CAD build for the part. Positions are in the model's coordinates, mm. Face numbers are marked on the shaded views. A direction names the side the tool comes from. Give positions to 0.01 mm unless a question says otherwise; leave off trailing zeros. Write each loop counter-clockwise with the first axis right and the second up, starting at its lowest first coordinate (ties: lowest second). Pieces come first, ordered by that corner, then holes. Notation, with made-up numbers: (60.5, 35.5) -> (93.5, 35.5) arc R22 ccw to (93.5, 73.5) -> close; hole circle Ø7 at (-30, 13). An arc over 180 degrees is marked (long way). Answer as a JSON object with one key per item and string values.
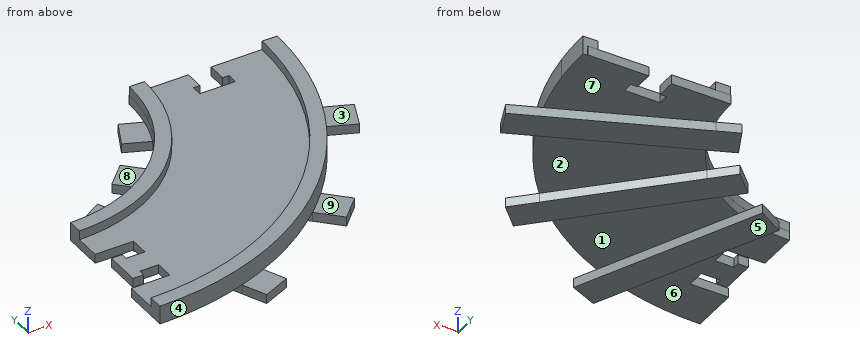
```python
from build123d import *

# Parameters (mm, degrees)
F1_DEPTH  = 3.175
F4_DEPTH  = 3.175
F6_DEPTH  = 6.35
F7_DEPTH  = 3.175
F9_DEPTH  = 25.4
F11_DEPTH = 3.175
F13_DEPTH = 3.175
F14_DEPTH = 25.4


with BuildPart() as f1:
    # F0 (on Top) → F1 (new body)
    with BuildSketch(Plane.XY):
        with BuildLine():
            Line((0, -51.2956328023), (0, -102.09075941))
            ThreePointArc((0, -102.09075941), (72.1890682753, -72.1890682753), (102.09075941, 0))
            Line((102.09075941, 0), (51.2956328023, 0))
            ThreePointArc((51.2956328023, 0), (36.2714897998, -36.2714897998), (0, -51.2956328023))
        make_face()
    extrude(amount=F1_DEPTH)

    # F3 (on face) → F4 (join)
    with BuildSketch(Plane.XY.offset(3.175)):
        with BuildLine():
            ThreePointArc((0, -56.3756328023), (39.8635922482, -39.8635922482), (56.3756328023, 0))
            Line((56.3756328023, 0), (51.3330261441, 0))
            ThreePointArc((51.3330261441, 0), (36.2979308853, -36.2979308853), (0, -51.3330261441))
            Line((0, -51.3330261441), (0, -56.3756328023))
        make_face()
        with BuildLine():
            Line((102.09075941, 0), (97.01075941, 0))
            ThreePointArc((97.01075941, 0), (68.5969658269, -68.5969658269), (0, -97.01075941))
            Line((0, -97.01075941), (0, -102.09075941))
            ThreePointArc((0, -102.09075941), (72.1890682753, -72.1890682753), (102.09075941, 0))
        make_face()
    extrude(amount=F4_DEPTH)

    # F5 (on Top) → F6 (join)
    with BuildSketch(Plane.XY):
        with BuildLine():
            ThreePointArc((54.7619331998, -13.660392724), (56.0189261095, -6.8815386855), (56.4400182242, 0))
            Line((56.4400182242, 0), (51.3051767249, 0))
            ThreePointArc((51.3051767249, 0), (50.8400637591, -6.8926827684), (49.4531579316, -13.660392724))
            Line((49.4531579316, -13.660392724), (54.7619331998, -13.660392724))
        make_face()
        with BuildLine():
            Line((102.1051767249, 0), (97.1390098326, 0))
            ThreePointArc((97.1390098326, 0), (96.8973822865, -6.8472284381), (96.1737017167, -13.660392724))
            Line((96.1737017167, -13.660392724), (101.1872560388, -13.660392724))
            ThreePointArc((101.1872560388, -13.660392724), (101.8754380952, -6.8455990928), (102.1051767249, 0))
        make_face()
    extrude(amount=F6_DEPTH)

    # F2 (on Top) → F7 (join)
    with BuildSketch(Plane.XY):
        Polygon((65.3862244444, -13.4132344524), (65.3862244444, 0.2373858813), (51.3049019501, 0.2373858813), (51.3049019501, -13.4632168472), align=None)
        Polygon((100.5855267867, 0.2373858813), (85.8938746733, 0.2373858813), (85.9641355587, -13.4132344524), (100.5855267867, -13.4132344524), align=None)
    extrude(amount=F7_DEPTH)

    # F8 (on face) → F9 (cut)
    with BuildSketch(Plane.XY.offset(3.175)):
        Polygon((0, -85.8303158734), (13.2304336887, -85.8303158734), (13.2304336887, -79.5142199461), (6.7552071823, -79.5142199461), (6.7552071823, -81.7240199461), (3.0578118576, -81.7240199461), (3.0578118576, -69.5130521654), (6.7552071823, -69.5130521654), (6.7552071823, -71.7228521654), (13.2304336887, -71.7228521654), (13.2304336887, -65.2524047592), (0, -65.2524047592), align=None)
    extrude(amount=-F9_DEPTH, mode=Mode.SUBTRACT)

    # F10 (on face) → F11 (join)
    with BuildSketch(Plane(origin=(0, 0, 0), x_dir=(1, 0, 0), z_dir=(0, 0, -1))):
        with BuildLine():
            ThreePointArc((39.6434592285, 32.5520826521), (37.980845771, 34.4774897449), (36.2248193412, 36.3181002847))
            Line((36.2248193412, 36.3181002847), (29.0498583475, 29.1246633635))
            Line((29.0498583475, 29.1246633635), (32.646576808, 25.5371828667))
            Line((32.646576808, 25.5371828667), (39.6434592285, 32.5520826521))
        make_face()
        with BuildLine():
            Line((29.0498583475, 29.1246633635), (36.2248193412, 36.3181002847))
            ThreePointArc((36.2248193412, 36.3181002847), (34.3796988436, 38.0693873344), (32.4500223073, 39.7270436459))
            Line((32.4500223073, 39.7270436459), (25.4531398869, 32.7121438604))
            Line((25.4531398869, 32.7121438604), (29.0498583475, 29.1246633635))
        make_face()
        with BuildLine():
            Line((36.2248193412, 36.3181002847), (72.0961827352, 72.2818344532))
            ThreePointArc((72.0961827352, 72.2818344532), (70.2749350461, 74.0537417095), (68.4101530773, 75.7797737714))
            Line((68.4101530773, 75.7797737714), (32.4500223073, 39.7270436459))
            ThreePointArc((32.4500223073, 39.7270436459), (34.3796988436, 38.0693873344), (36.2248193412, 36.3181002847))
        make_face()
        with BuildLine():
            ThreePointArc((75.6035899985, 68.6048127777), (73.8727679087, 70.4651496728), (72.0961827352, 72.2818344532))
            Line((72.0961827352, 72.2818344532), (36.2248193412, 36.3181002847))
            ThreePointArc((36.2248193412, 36.3181002847), (37.980845771, 34.4774897449), (39.6434592285, 32.5520826521))
            Line((39.6434592285, 32.5520826521), (75.6035899985, 68.6048127777))
        make_face()
        with BuildLine():
            Line((79.271143729, 79.4752713743), (72.0961827352, 72.2818344532))
            ThreePointArc((72.0961827352, 72.2818344532), (73.8727679087, 70.4651496728), (75.6035899985, 68.6048127777))
            Line((75.6035899985, 68.6048127777), (82.8785053866, 75.8984614814))
            Line((82.8785053866, 75.8984614814), (79.271143729, 79.4752713743))
        make_face()
        with BuildLine():
            ThreePointArc((68.4101530773, 75.7797737714), (70.2749350461, 74.0537417095), (72.0961827352, 72.2818344532))
            Line((72.0961827352, 72.2818344532), (79.271143729, 79.4752713743))
            Line((79.271143729, 79.4752713743), (75.7328631666, 83.1213402502))
            Line((75.7328631666, 83.1213402502), (68.4101530773, 75.7797737714))
        make_face()
        with BuildLine():
            Line((20.0341812257, 47.2215366883), (40.6881574418, 93.6322433828))
            ThreePointArc((40.6881574418, 93.6322433828), (35.9596571955, 95.5480309127), (31.1413521737, 97.2251991086))
            Line((31.1413521737, 97.2251991086), (10.2418471319, 50.2627746142))
            ThreePointArc((10.2418471319, 50.2627746142), (15.2141958482, 48.9874493037), (20.0341812257, 47.2215366883))
        make_face()
        with BuildLine():
            ThreePointArc((31.1413521737, 97.2251991086), (35.9596571955, 95.5480309127), (40.6881574418, 93.6322433828))
            Line((40.6881574418, 93.6322433828), (44.0618023276, 101.2130230665))
            Line((44.0618023276, 101.2130230665), (34.7585338749, 105.353220427))
            Line((34.7585338749, 105.353220427), (31.1413521737, 97.2251991086))
        make_face()
        with BuildLine():
            Line((16.5176168084, 39.3196083605), (20.0341812257, 47.2215366883))
            ThreePointArc((20.0341812257, 47.2215366883), (15.2141958482, 48.9874493037), (10.2418471319, 50.2627746142))
            Line((10.2418471319, 50.2627746142), (7.7137911807, 44.5820833017))
            Line((7.7137911807, 44.5820833017), (16.5176168084, 39.3196083605))
        make_face()
        with BuildLine():
            ThreePointArc((50.2968928634, 10.0729594896), (49.0339423103, 15.0636796999), (47.2771132537, 19.902675875))
            Line((47.2771132537, 19.902675875), (38.7149937451, 16.3121093065))
            Line((38.7149937451, 16.3121093065), (43.1567628434, 7.0787111473))
            Line((43.1567628434, 7.0787111473), (50.2968928634, 10.0729594896))
        make_face()
        with BuildLine():
            ThreePointArc((97.6098508897, 29.9138791566), (95.9858944102, 34.7740022313), (94.1201154327, 39.5465172658))
            Line((94.1201154327, 39.5465172658), (47.2771132537, 19.902675875))
            ThreePointArc((47.2771132537, 19.902675875), (49.0339423103, 15.0636796999), (50.2968928634, 10.0729594896))
            Line((50.2968928634, 10.0729594896), (97.6098508897, 29.9138791566))
        make_face()
        with BuildLine():
            Line((104.0109246969, 43.6942763627), (94.1201154327, 39.5465172658))
            ThreePointArc((94.1201154327, 39.5465172658), (95.9858944102, 34.7740022313), (97.6098508897, 29.9138791566))
            Line((97.6098508897, 29.9138791566), (107.9681979582, 34.2577025116))
            Line((107.9681979582, 34.2577025116), (104.0109246969, 43.6942763627))
        make_face()
    extrude(amount=F11_DEPTH)

    # F12 (on face) → F13 (join)
    with BuildSketch(Plane(origin=(0, 0, 0), x_dir=(1, 0, 0), z_dir=(0, 0, -1))):
        Polygon((65.3862244444, 0), (65.3862244444, -0.2373858813), (85.8938746733, -0.2373858813), (85.8950965183, 0), align=None)
    extrude(amount=-F13_DEPTH)

    # F2 (on Top) → F14 (cut)
    with BuildSketch(Plane.XY):
        Polygon((81.7886919434, -6.2948371671), (79.5788919434, -6.2948371671), (79.5788919434, 0.2373858813), (71.7875241627, 0.2373858813), (71.7875241627, -6.2948371671), (69.5777241627, -6.2948371671), (69.5777241627, -9.9109848417), (81.7886919434, -9.9109848417), align=None)
    extrude(amount=F14_DEPTH, mode=Mode.SUBTRACT)


solid = f1.part
```
1) Slice it at A-A (y = -28.5). List the corners of the cut face in (x, z) (3 decimals).
Model answer:
{"outline": "(29.676, -3.175) -> (35.602, -3.175) -> (35.602, 0) -> (29.676, 0) -> close; (42.65, 0) -> (67.778, 0) -> (67.778, -3.175) -> (94.238, -3.175) -> (94.238, 0) -> (98.032, 0) -> (98.032, 6.35) -> (92.73, 6.35) -> (92.73, 3.175) -> (48.641, 3.175) -> (48.641, 6.35) -> (42.695, 6.35) -> (42.695, 3.175) -> (42.65, 3.175) -> close"}
2) Slice it at D-D (y = -74). List the corners of the cut face in (x, z) (3 decimals), then the cut area to 3 significant figures.
Model answer:
{"outline": "(3.058, 0) -> (20.806, 0) -> (20.806, -3.175) -> (31.951, -3.175) -> (31.951, 0) -> (66.635, 0) -> (66.635, -3.175) -> (80.985, -3.175) -> (80.985, 0) -> (70.332, 0) -> (70.332, 6.35) -> (62.73, 6.35) -> (62.73, 3.175) -> (3.058, 3.175) -> close", "area": "319 mm2"}
3) 3-axis set-ups, long thin cutter, end or side, ignore diameter. For the marked faces 5, 6, 7, 8 and 9: which of +Z, -Z, +X, -X, +Y, -Y reach the whole face in a straight line?
Model answer:
{"face 5": "-Z, +X, -X, +Y, -Y", "face 6": "-Z, -X, -Y", "face 7": "-Z, +X, +Y", "face 8": "+Z, -X, +Y", "face 9": "+Z, +X, -Y"}
4) Pin check, flat tips, straight feed: pin 1 (2 mm diameter, centred on y = -15, z = 1.5, fed in from -X); pin 2 (1.6 mm diameter, centred on y = -81, z = 2.5, fed in from -X); pin 3 (12 mm diameter, centred on x = 12.5, y = -43.5, fed in from +Z). Stop position of each tip, or through.
Model answer:
{"pin 1": "stops at x = 48.74", "pin 2": "stops at x = 3.06", "pin 3": "stops at z = 0"}
5) Mould opens along Y. For the marked faces 1, 2, 3 and 4 say: released by +Y, released by -Y, zero draft, split by the parting line, or undercut.
Model answer:
{"face 1": "undercut", "face 2": "undercut", "face 3": "zero draft", "face 4": "released by -Y"}
6) Slice it at C-C (y = -12). List the corners of the cut face in (x, z) (3 decimals).
Model answer:
{"outline": "(40.789, -3.175) -> (54.892, -3.175) -> (54.892, 0) -> (101.398, 0) -> (101.398, 6.35) -> (96.266, 6.35) -> (96.266, 3.175) -> (55.15, 3.175) -> (55.15, 6.35) -> (49.882, 6.35) -> (49.882, 3.175) -> (49.872, 3.175) -> (49.872, 0) -> (40.789, 0) -> close"}
7) Wall check: probe 1 along Z at (x, y) = (35, -89) (3 decimals); probe 2 along Z at (x, y) = (72, -75.5) (3 decimals); probe 3 along X at (y, z) = (-80.5, 2.75). Give the ranges that are in metal, low to high.
Model answer:
{"probe 1": "z = -3.175 to 3.175", "probe 2": "z = -3.175 to 0", "probe 3": "x = 3.06 to 6.76, 13.23 to 62.79"}
8) Slice it at B-B (x = 37.5). List the corners of the cut face in (y, z) (3 decimals).
Model answer:
{"outline": "(-104.133, -3.175) -> (-86.468, -3.175) -> (-86.468, 0) -> (-44.79, 0) -> (-44.79, -3.175) -> (-30.403, -3.175) -> (-30.403, 0) -> (-35, 0) -> (-35, 3.175) -> (-35.055, 3.175) -> (-35.055, 6.35) -> (-42.095, 6.35) -> (-42.095, 3.175) -> (-89.47, 3.175) -> (-89.47, 6.35) -> (-94.954, 6.35) -> (-94.954, 0) -> (-104.133, 0) -> close"}
